from build123d import *

# Parameters (mm, degrees)
SKETCH1_R                       = 2.5
BOSS_EXTRUDE1_DEPTH             = 15
SKETCH2_R                       = 1
CUT_EXTRUDE1_DEPTH              = 16.411035007
TAP_DRILL_FOR_M4X0_7_TAP1_D     = 3.3
TAP_DRILL_FOR_M4X0_7_TAP1_DEPTH = 9
TAP_DRILL_FOR_M4X0_7_TAP1_TIP   = 0.991420021
SKETCH5_W                       = 3
SKETCH5_H                       = 1.793791595
CHAMFER1_SIZE                   = 0.5
CHAMFER1_SIZE2                  = 0.866025404
CHAMFER2_SIZE                   = 1.21
CHAMFER2_SIZE2                  = 0.698593826


with BuildPart() as part:
    # Sketch1 → Boss-Extrude1 (new body)
    with BuildSketch(Plane.XY):
        Circle(SKETCH1_R)
    extrude(amount=BOSS_EXTRUDE1_DEPTH)

    # Sketch2 → Cut-Extrude1 (cut, through all)
    with BuildSketch(Plane(origin=(0, 0, 0), x_dir=(-1, 0, 0), z_dir=(0, 0, -1))):
        Circle(SKETCH2_R)
    extrude(amount=-CUT_EXTRUDE1_DEPTH, mode=Mode.SUBTRACT)

    # Tap Drill for M4x0.7 Tap1
    with Locations(Plane(origin=(0, 0, 0), x_dir=(-1, 0, 0), z_dir=(0, 0, -1))):
        with Locations((0, 0)):
            Hole(TAP_DRILL_FOR_M4X0_7_TAP1_D / 2, depth=TAP_DRILL_FOR_M4X0_7_TAP1_DEPTH)
            with Locations((0, 0, -(TAP_DRILL_FOR_M4X0_7_TAP1_DEPTH + TAP_DRILL_FOR_M4X0_7_TAP1_TIP / 2))):  # 118° drill point
                Cone(0, TAP_DRILL_FOR_M4X0_7_TAP1_D / 2, TAP_DRILL_FOR_M4X0_7_TAP1_TIP, mode=Mode.SUBTRACT)

    # Sketch5 → Cut-Revolve1 (revolve, cut)
    with BuildSketch(Plane(origin=(0, 0, 0), x_dir=(0, 0, -1), z_dir=(1, 0, 0)), mode=Mode.PRIVATE) as cut_revolve1_sk:
        with Locations((-12.5, 2.896895798)):
            Rectangle(SKETCH5_W, SKETCH5_H)
    revolve(cut_revolve1_sk.sketch.rotate(Axis((0, 0, 0), (0, 0, 1)), 90), axis=Axis((0, 0, 0), (0, 0, 1)), mode=Mode.SUBTRACT)

    # Chamfer1
    chamfer1_edges = [part.edges().sort_by_distance(p)[0] for p in [
        (-1.65, 0, 0),
    ]]
    chamfer1_side = [part.faces().sort_by_distance(p)[0] for p in [
        (-2.429289322, 0, 0),
    ]]
    chamfer(chamfer1_edges, length=CHAMFER1_SIZE, length2=CHAMFER1_SIZE2, reference=chamfer1_side[0])

    # Chamfer2
    chamfer2_edges = [part.edges().sort_by_distance(p)[0] for p in [
        (1, 0, 15),
    ]]
    chamfer2_side = [part.faces().sort_by_distance(p)[0] for p in [
        (1, 0, 12.195279701),
    ]]
    chamfer(chamfer2_edges, length=CHAMFER2_SIZE, length2=CHAMFER2_SIZE2, reference=chamfer2_side[0])


solid = part.part
Can you work these out from the model? Positions are in its coordinate system, mm. A direction names the side the tool comes from. Give positions to 0.01 mm unless a question says otherwise; leave off trailing zeros. Order: outer loops, then holes, each group sorted by start corner. A loop starts at its lowest first (then second) coordinate and runs counter-clockwise, first axis right, second up. Notation, with made-up numbers: M 39,10 L 76,10 A35 ccw 76,48 Z; hole C 44,76 d5. An arc over 180 degrees is marked long. Use a Markdown table: item, result. Add a question column.
Item 1: For faces 4 (the cylindrical face through (-1.216, 1.115, 4.99)), 5 (the cylindrical face through (-0.54, -2.44, 5.42)), 6 (the flat face through (-1, -2, 14)), which set-ups out of +Z, -Z, +X, -X, +Y, -Y let a thin tool reach every point of the face, with its end or its side?
Item 2: Suppose I cut it at C-C (z = 10.5). List the corners of the cut face in (x, y) for me, then the cut area to 3 significant figures.
Item 3: Will these pins go through, and if not, where does the flat tip stop? pin 1 (2.5 mm diameter, centred on x = 0, y = 0, fed in from -Z); pin 2 (1.5 mm diameter, centred on x = 0.5, y = 0.5, fed in from +Z); pin 3 (2 mm diameter, centred on y = -1.5, z = 8.5, fed in from -X).
Item 4: If I drill on L1, parallel to Z at x = 1.8, y = -1.4; L2, parallel to X at y = 0, z = 5.25, over which ranges is the centre line in solid material (lowest first)? Write a range as [from, to].
Item 5: Suppose I cut it at A-A (y = 0). List the corners of the cut face in (x, z) for me.
Item 6: We'd pull the mould along Z, two halves only. Please class faces 1 (the flat face through (2, -1, 15)), 2 (the cylindrical face through (1.474, -1.352, 12.479)), 3 (the cylindrical face through (0, -1, 12)): +Z half, -Z half, draft (parallel to the pull), parting line (faces both ways), or undercut.
Answer sheet:
| question | item | result |
|---|---|---|
| 1 | face 4 | -Z |
| 1 | face 5 | +Z, -Z |
| 1 | face 6 | none |
| 2 | outline | C 0,0 d5; hole C 0,0 d2 |
| 2 | area | 16.5 mm² |
| 3 | pin 1 | stops at z = 9.24 |
| 3 | pin 2 | stops at z = 14.58 |
| 3 | pin 3 | stops at x = -2.45 |
| 4 | L1 | z = [0, 11], [14, 15] |
| 4 | L2 | x = [-2.5, -1.65], [1.65, 2.5] |
| 5 | outline | M -2.5,0 L -2.15,0 L -1.65,0.87 L -1.65,9 L -1,9.39 L -1,13.79 L -1.7,15 L -2.5,15 L -2.5,14 L -2,14 L -2,11 L -2.5,11 Z; M 1,9.39 L 1.65,9 L 1.65,0.87 L 2.15,0 L 2.5,0 L 2.5,11 L 2,11 L 2,14 L 2.5,14 L 2.5,15 L 1.7,15 L 1,13.79 Z |
| 6 | face 1 | +Z half |
| 6 | face 2 | undercut |
| 6 | face 3 | draft |
